Input: part model. Units: mm. Frame: model coordinates. Coordinates: 2 decimals unless noted, no trailing zeros. Order: outer loops, then holes, each group sorted by start corner. A loop starts at its lowest first (then second) coordinate and runs counter-clockwise, first axis right, second up. Notation, with made-up numbers: (-14, -39.75) - (17, -39.75) arc R23 cw to (17, -29.75) - close; hole circle Ø9 at (88.5, -19). An arc over 180 degrees is marked (long way). Use a Markdown table: item, result. Add a question column.
from build123d import *

# Parameters (mm, degrees)
BOSS_EXTRUDE1_DEPTH = 6.35
CHAMFER9_SIZE       = 2.54
CHAMFER10_SIZE      = 2.54
CHAMFER11_SIZE      = 2.54
CHAMFER12_SIZE      = 2.54
CHAMFER13_SIZE      = 2.54
FILLET1_R           = 8.89
SKETCH2_R           = 2.159
CUT_EXTRUDE1_DEPTH  = 7.35


with BuildPart() as part:
    # Sketch1 → Boss-Extrude1 (new body)
    with BuildSketch(Plane(origin=(0, 0, 0), x_dir=(1, 0, 0), z_dir=(0, 1, 0))):
        Polygon((-45.908148148, -30.432962963), (-20.508148148, -30.432962963), (-20.508148148, 20.367037037), (30.291851852, 20.367037037), (30.291851852, 45.767037037), (-20.508148148, 45.767037037), (-45.908148148, 45.767037037), (-45.908148148, 20.367037037), align=None)
    extrude(amount=BOSS_EXTRUDE1_DEPTH)

    # Chamfer9
    chamfer9_edges = [part.edges().sort_by_distance(p)[0] for p in [
        (-20.508148148, 3.175, 30.432962963),
    ]]
    chamfer(chamfer9_edges, length=CHAMFER9_SIZE)

    # Chamfer10
    chamfer10_edges = [part.edges().sort_by_distance(p)[0] for p in [
        (30.291851852, 3.175, -20.367037037),
    ]]
    chamfer(chamfer10_edges, length=CHAMFER10_SIZE)

    # Chamfer11
    chamfer11_edges = [part.edges().sort_by_distance(p)[0] for p in [
        (30.291851852, 3.175, -45.767037037),
    ]]
    chamfer(chamfer11_edges, length=CHAMFER11_SIZE)

    # Chamfer12
    chamfer12_edges = [part.edges().sort_by_distance(p)[0] for p in [
        (-45.908148148, 3.175, 30.432962963),
    ]]
    chamfer(chamfer12_edges, length=CHAMFER12_SIZE)

    # Chamfer13
    chamfer13_edges = [part.edges().sort_by_distance(p)[0] for p in [
        (-45.908148148, 3.175, -45.767037037),
    ]]
    chamfer(chamfer13_edges, length=CHAMFER13_SIZE)

    # Fillet1
    fillet1_edges = [part.edges().sort_by_distance(p)[0] for p in [
        (-20.508148148, 3.175, -20.367037037),
    ]]
    fillet(fillet1_edges, radius=FILLET1_R)

    # Sketch2 → Cut-Extrude1 (cut, through all)
    with BuildSketch(Plane(origin=(0, 6.35, 0), x_dir=(1, 0, 0), z_dir=(0, 1, 0))):
        with Locations((-33.208148148, 33.067037037)):
            Circle(SKETCH2_R)
        with Locations((-20.508148148, 33.067037037)):
            Circle(SKETCH2_R)
        with Locations((-7.808148148, 33.067037037)):
            Circle(SKETCH2_R)
        with Locations((4.891851852, 33.067037037)):
            Circle(SKETCH2_R)
        with Locations((17.591851852, 33.067037037)):
            Circle(SKETCH2_R)
        with Locations((-33.208148148, 20.367037037)):
            Circle(SKETCH2_R)
        with Locations((-33.208148148, 7.667037037)):
            Circle(SKETCH2_R)
        with Locations((-33.208148148, -5.032962963)):
            Circle(SKETCH2_R)
        with Locations((-33.208148148, -17.732962963)):
            Circle(SKETCH2_R)
    extrude(amount=-CUT_EXTRUDE1_DEPTH, mode=Mode.SUBTRACT)


solid = part.part
1) Cut plane B-B (y = 4.5). State how many separate pieces and enclosed holes the cut face has, and give its area (3 significant figures).
2) Cut plane D-D (z = -16.5). Return the cut outline in (x, y).
3) Cut plane A-A (x = -7). Return the cut outline in (y, z) (3 decimals), and give its area (3 significant figures).
4) Cut plane C-C (z = -4). Return the cut outline in (x, y), and give its area (3 significant figures).
5) Material intervals for L1, parallel to Z at x = -33, y = 5; L2, parallel to Z at x = 5, y = 4; L3, parallel to X at y = 2.75, z = -35, sorted ascending.
6) Pull-direction query (X, two-part tool) for faces 1 (the cylindrical face through (4.42, 3.22, -30.96)), 2 (the flat face through (29.004, 3.131, -44.515)), 3 (the flat face through (-44.6, 3.1, 29.2)), 4 (the flat face through (-17, 6.35, -25)); classes: pulls with the +X half, pulls with the -X half, needs draft (parallel to the pull), parting line crosses it, or undercut.
7) Contact query for flat-ended pins moving along their axis: P1, Ø3, axis at y = 3, z = 1.5, coming from the +X side; P2, Ø3, axis at x = 9, y = 4, coming from the +Z side. Output: stop coordinate, or through.
Computed:
| question | item | result |
|---|---|---|
| 1 | separate pieces | 1 |
| 1 | enclosed holes | 9 |
| 1 | area | 3,090 mm2 |
| 2 | outline | (-45.91, 0) - (-18.95, 0) - (-18.95, 6.35) - (-45.91, 6.35) - close |
| 3 | outline | (0, -45.767) - (6.35, -45.767) - (6.35, -35.069) - (0, -35.069) - close; (0, -31.065) - (6.35, -31.065) - (6.35, -20.367) - (0, -20.367) - close |
| 3 | area | 136 mm2 |
| 4 | outline | (-45.91, 0) - (-20.51, 0) - (-20.51, 6.35) - (-45.91, 6.35) - close |
| 4 | area | 161 mm2 |
| 5 | L1 | z = -45.77 to -35.22, -30.92 to -22.52, -18.22 to -9.82, -5.52 to 2.88, 7.18 to 15.58, 19.88 to 30.43 |
| 5 | L2 | z = -45.77 to -35.22, -30.91 to -20.37 |
| 5 | L3 | x = -45.91 to -34.17, -32.25 to -21.47, -19.55 to -8.77, -6.85 to 3.93, 5.85 to 16.63, 18.55 to 30.29 |
| 6 | face 1 | undercut |
| 6 | face 2 | pulls with the +X half |
| 6 | face 3 | pulls with the -X half |
| 6 | face 4 | needs draft |
| 7 | P1 | stops at x = -20.51 |
| 7 | P2 | stops at z = -20.37 |
